from build123d import *

# Parameters (mm, degrees)
IZIM1_W                     = 78
IZIM1_H                     = 150
Y_KSEKLIK_EKSTR_ZYON1_DEPTH = 18
IZIM2_W                     = 73
IZIM2_H                     = 17
KES_EKSTR_ZYON1_DEPTH       = 143
IZIM3_W                     = 78
IZIM3_H                     = 150
Y_KSEKLIK_EKSTR_ZYON2_DEPTH = 5
IZIM4_W                     = 73
IZIM4_H                     = 17
KES_EKSTR_ZYON2_DEPTH       = 148
IZIM6_W                     = 58
IZIM6_H                     = 130
IZIM6_H_2                   = 10
KES_EKSTR_ZYON3_DEPTH       = 10
IZIM7_W                     = 45.739377618
IZIM7_H                     = 2.329706958
KES_EKSTR_ZYON5_DEPTH       = 147
IZIM8_W                     = 94
IZIM8_H                     = 16.552930253
Y_KSEKLIK_EKSTR_ZYON4_DEPTH = 3
IZIM10_W                    = 73
IZIM10_H                    = 17
KES_EKSTR_ZYON7_DEPTH       = 146
IZIM11_R                    = 1.5
KES_EKSTR_ZYON8_DEPTH       = 146


with BuildPart() as part:
    # Çizim1 → Yükseklik-Ekstrüzyon1 (new body)
    with BuildSketch(Plane(origin=(0, 0, 0), x_dir=(1, 0, 0), z_dir=(0, 1, 0))):
        with Locations((8.016202101, 19.801973492)):
            Rectangle(IZIM1_W, IZIM1_H)
    extrude(amount=Y_KSEKLIK_EKSTR_ZYON1_DEPTH)

    # Çizim2 → Kes-Ekstrüzyon1 (cut)
    with BuildSketch(Plane(origin=(0, 0, -94.801973492), x_dir=(-1, 0, 0), z_dir=(0, 0, -1))):
        with Locations((-8.016202101, 10)):
            Rectangle(IZIM2_W, IZIM2_H)
    extrude(amount=-KES_EKSTR_ZYON1_DEPTH, mode=Mode.SUBTRACT)

    # Çizim3 → Yükseklik-Ekstrüzyon2 (add)
    with BuildSketch(Plane(origin=(0, 18, 0), x_dir=(1, 0, 0), z_dir=(0, 1, 0))):
        with Locations((8.016202101, 19.801973492)):
            Rectangle(IZIM3_W, IZIM3_H)
    extrude(amount=Y_KSEKLIK_EKSTR_ZYON2_DEPTH)

    # Çizim4 → Kes-Ekstrüzyon2 (cut)
    with BuildSketch(Plane(origin=(0, 0, -94.801973492), x_dir=(-1, 0, 0), z_dir=(0, 0, -1))):
        with Locations((-8.016202101, 10)):
            Rectangle(IZIM4_W, IZIM4_H)
    extrude(amount=-KES_EKSTR_ZYON2_DEPTH, mode=Mode.SUBTRACT)

    # Çizim6 → Kes-Ekstrüzyon3 (cut)
    with BuildSketch(Plane(origin=(0, 23, 0), x_dir=(1, 0, 0), z_dir=(0, 1, 0))):
        with Locations((8.016202101, 19.801973492)):
            Rectangle(IZIM6_W, IZIM6_H)
        with Locations((8.016202101, 89.801973492)):
            Rectangle(IZIM6_W, IZIM6_H_2)
    extrude(amount=-KES_EKSTR_ZYON3_DEPTH, mode=Mode.SUBTRACT)

    # Çizim7 → Kes-Ekstrüzyon5 (cut)
    with BuildSketch(Plane(origin=(47.016202101, 0, 0), x_dir=(0, 0, -1), z_dir=(1, 0, 0))):
        with Locations((24.733454375, 16.908564322)):
            Rectangle(IZIM7_W, IZIM7_H)
    extrude(amount=-KES_EKSTR_ZYON5_DEPTH, mode=Mode.SUBTRACT)

    # Çizim8 → Yükseklik-Ekstrüzyon4 (add)
    with BuildSketch(Plane.XZ):
        with Locations((8.016202101, 41.439700866)):
            Rectangle(IZIM8_W, IZIM8_H)
        with Locations((8.016202101, -81.04364785)):
            Rectangle(IZIM8_W, IZIM8_H)
    extrude(amount=-Y_KSEKLIK_EKSTR_ZYON4_DEPTH)

    # Çizim10 → Kes-Ekstrüzyon7 (cut)
    with BuildSketch(Plane(origin=(0, 0, -94.801973492), x_dir=(-1, 0, 0), z_dir=(0, 0, -1))):
        with Locations((-8.016202101, 10)):
            Rectangle(IZIM10_W, IZIM10_H)
    extrude(amount=-KES_EKSTR_ZYON7_DEPTH, mode=Mode.SUBTRACT)

    # Çizim11 → Kes-Ekstrüzyon8 (cut)
    with BuildSketch(Plane(origin=(0, 3, 0), x_dir=(1, 0, 0), z_dir=(0, 1, 0))):
        with Locations((-34.983797899, -41.439700866)):
            Circle(IZIM11_R)
        with Locations((51.016202101, -41.439700866)):
            Circle(IZIM11_R)
        with Locations((51.016202101, 81.043647849)):
            Circle(IZIM11_R)
        with Locations((-34.983797899, 81.043647849)):
            Circle(IZIM11_R)
    extrude(amount=-KES_EKSTR_ZYON8_DEPTH, mode=Mode.SUBTRACT)


solid = part.part
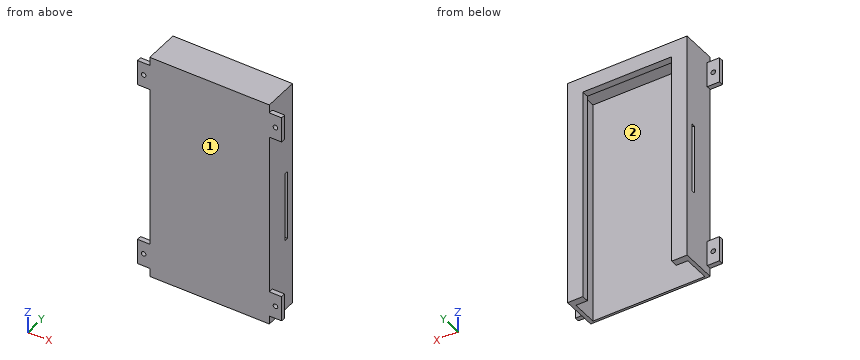
Read the model definition and answer for the solid it produces. Units are mm, in the model's axes. Face numbers are marked on the shaded views. Give positions to 0.01 mm unless a question says otherwise; leave off trailing zeros. Loops run counter-clockwise (first coordinate to the right, second up) from the corner with the lowest first, then second, coordinate; pieces in that order, holes last. Notation, with made-up numbers: (-37.75, -35.75) -> (8.25, -35.75) arc R10 ccw to (8.25, -22.75) -> close; hole circle Ø4 at (10.25, 50.5). An arc over 180 degrees is marked (long way). Use a Markdown table: item, result.
Q1. Section A-A, the plane z = -33 is taken. Determine the outline of the cut face in (x, y).
Solved:
| item | result |
|---|---|
| outline | (-30.98, 0) -> (47.02, 0) -> (47.02, 15.74) -> (44.52, 15.74) -> (44.52, 1.5) -> (-28.48, 1.5) -> (-28.48, 15.74) -> (-30.98, 15.74) -> close; (-30.98, 18.07) -> (-28.48, 18.07) -> (-28.48, 18.5) -> (-20.98, 18.5) -> (-20.98, 23) -> (-30.98, 23) -> close; (37.02, 18.5) -> (44.52, 18.5) -> (44.52, 18.07) -> (47.02, 18.07) -> (47.02, 23) -> (37.02, 23) -> close |
Q2. Section B-B, the plane z = 15 is taken. Determine the outline of the cut face in (x, y).
Solved:
| item | result |
|---|---|
| outline | (-30.98, 0) -> (47.02, 0) -> (47.02, 23) -> (37.02, 23) -> (37.02, 18.5) -> (44.52, 18.5) -> (44.52, 1.5) -> (-28.48, 1.5) -> (-28.48, 18.5) -> (-20.98, 18.5) -> (-20.98, 23) -> (-30.98, 23) -> close |
Q3. Section D-D, the plane y = 10.75 is taken. Determine the outline of the cut face in (x, z), then the cut area to 3 significant figures.
Solved:
| item | result |
|---|---|
| outline | (-30.98, -94.8) -> (-28.48, -94.8) -> (-28.48, 53.2) -> (44.52, 53.2) -> (44.52, -94.8) -> (47.02, -94.8) -> (47.02, 55.2) -> (-30.98, 55.2) -> close |
| area | 896 mm^2 |
Q4. Determine the mould class of the marked faces 1 and 2 for opening direction X: pulls with the +X half, pulls with the -X half, needs draft (parallel to the pull), parting line crosses it, or undercut.
Solved:
| item | result |
|---|---|
| face 1 | needs draft |
| face 2 | undercut |
Q5. Section C-C, the plane x = 10.5 is taken. Determine the outline of the cut face in (y, z).
Solved:
| item | result |
|---|---|
| outline | (0, -94.8) -> (1.5, -94.8) -> (1.5, 53.2) -> (18.5, 53.2) -> (18.5, 45.2) -> (23, 45.2) -> (23, 55.2) -> (0, 55.2) -> close |
Q6. Find the intervals of material crossed by line 1 along X through (y, z) = (14, 17.5); line 2 along X through (y, z) = (22, -40); line 3 along Y through (x, z) = (36, 47), in increasing order.
Solved:
| item | result |
|---|---|
| line 1 | x = -30.98 to -28.48, 44.52 to 47.02 |
| line 2 | x = -30.98 to -20.98, 37.02 to 47.02 |
| line 3 | y = 0 to 1.5, 18.5 to 23 |
Q7. Each of these flat-tipped pins is pushed along its axis until it touches: pin 1 (3.5 mm diameter, centred on y = 20, z = 7.5, fed in from +X); pin 2 (3.5 mm diameter, centred on y = 21, z = -45, fed in from -X); pin 3 (0.9 mm diameter, centred on x = -35.5, y = 1.5, fed in from -Z). Where does it stop, or does it pass through?
Solved:
| item | result |
|---|---|
| pin 1 | stops at x = 47.02 |
| pin 2 | stops at x = -30.98 |
| pin 3 | stops at z = -89.32 |
